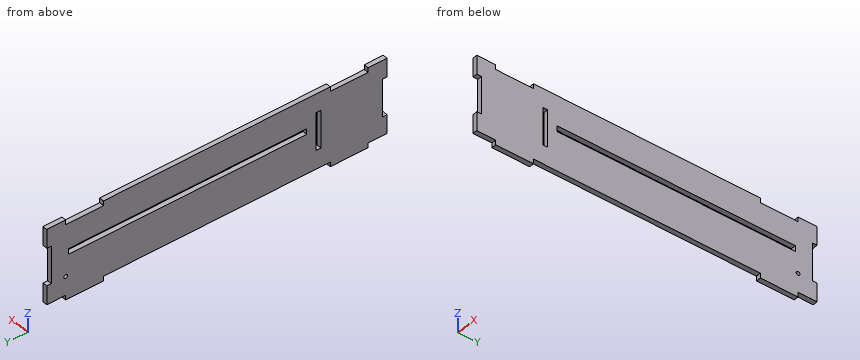
from build123d import *

# Parameters (mm, degrees)
F0_W      = 457.2
F0_H      = 101.6
F1_DEPTH  = 6.35
F2_W      = 50.8
F2_H      = 6.35
F3_DEPTH  = 6.35
F4_R      = 2.54
F5_DEPTH  = 6.351
F6_W      = 6.35
F6_H      = 50.8
F7_DEPTH  = 25.4
F9_W      = 6.35
F9_H      = 50.8
F10_DEPTH = 25.4
F11_W     = 50.8
F11_H     = 6.35
F12_DEPTH = 25.4
F13_W     = 320.04
F13_H     = 7.62
F14_DEPTH = 25.4


with BuildPart() as f1:
    # F0 (on Right) → F1 (new body)
    with BuildSketch(Plane.YZ):
        with Locations((0, 50.8)):
            Rectangle(F0_W, F0_H)
    extrude(amount=F1_DEPTH)

    # F4 (on face) → F5 (cut, through all)
    with BuildSketch(Plane.YZ.offset(6.35)):
        with Locations((203.2, 25.4)):
            Circle(F4_R)
    extrude(amount=-F5_DEPTH, mode=Mode.SUBTRACT)

    # F6 (on face) → F7 (cut)
    with BuildSketch(Plane.YZ.offset(6.35)):
        with Locations((225.425, 50.8)):
            Rectangle(F6_W, F6_H)
        with Locations((-225.425, 50.8)):
            Rectangle(F6_W, F6_H)
    extrude(amount=-F7_DEPTH, mode=Mode.SUBTRACT)


with BuildPart() as f3:
    # F2 (on face) → F3 (new body)
    with BuildSketch(Plane.YZ.offset(6.35)):
        with Locations((177.8, -3.175)):
            Rectangle(F2_W, F2_H)
        with Locations((-177.8, -3.175)):
            Rectangle(F2_W, F2_H)
    extrude(amount=-F3_DEPTH)

    # F8: union F1
    add(f1.part)

    # F9 (on face) → F10 (cut)
    with BuildSketch(Plane.YZ.offset(6.35)):
        with Locations((-136.525, 50.8)):
            Rectangle(F9_W, F9_H)
    extrude(amount=-F10_DEPTH, mode=Mode.SUBTRACT)

    # F11 (on face) → F12 (cut)
    with BuildSketch(Plane.YZ.offset(6.35)):
        with Locations((-177.8, 98.425)):
            Rectangle(F11_W, F11_H)
        with Locations((177.8, 98.425)):
            Rectangle(F11_W, F11_H)
    extrude(amount=-F12_DEPTH, mode=Mode.SUBTRACT)

    # F13 (on face) → F14 (cut)
    with BuildSketch(Plane.YZ.offset(6.35)):
        with Locations((39.37, 57.15)):
            Rectangle(F13_W, F13_H)
    extrude(amount=-F14_DEPTH, mode=Mode.SUBTRACT)


solid = f3.part
The model under review builds one solid part; all positions refer to its coordinate system, in mm. Round coordinates to 2 decimals unless told otherwise and drop trailing zeros. Write each loop counter-clockwise with the first axis right and the second up, starting at its lowest first coordinate (ties: lowest second). Pieces come first, ordered by that corner, then holes. Notation, with made-up numbers: M -34,67 L 25,67 A29 ccw 25,87 Z; hole C 2.5,-24 d2. An arc over 180 degrees is marked long. Use a Markdown table: item, result. Add a question column.
Q1. We need section B-B, the plane z = 67. State the section outline as (x, y) points.
Q2. We need section C-C, the plane x = 1. Count the separate pieces of the cut face and the enclosed holes in it, plus the area to 3 significant figures.
Q3. Insertion check: pin 1 (1.9 mm diameter, centred on x = 4, z = -4, fed in from +Y); pin 2 (3 mm diameter, centred on x = 2, y = -219, fed in from -Z); pin 3 (1 mm diameter, centred on x = 1, z = 57.5, fed in from -Y). Each pin has a flat end and moves straight along its axis. Give the tip position at first contact, or say it passes through.
Q4. We need section A-A, the plane y = -96. State the section outline as (x, z) points.
Q5. To check wall thickness, follow line 1 (Y direction, x = 1, z = 48.5); line 2 (Z direction, x = 2.25, y = 90); line 3 (Y direction, x = 1.25, z = -0.5). State the ranges of each line that lie inside material, in increasing order.
Findings below:
| question | item | result |
|---|---|---|
| 1 | outline | M 0,-222.25 L 6.35,-222.25 L 6.35,-139.7 L 0,-139.7 Z; M 0,-133.35 L 6.35,-133.35 L 6.35,222.25 L 0,222.25 Z |
| 2 | separate pieces | 1 |
| 2 | enclosed holes | 3 |
| 2 | area | 43,000 mm² |
| 3 | pin 1 | stops at y = 203.2 |
| 3 | pin 2 | stops at z = 0 |
| 3 | pin 3 | stops at y = -222.25 |
| 4 | outline | M 0,0 L 6.35,0 L 6.35,53.34 L 0,53.34 Z; M 0,60.96 L 6.35,60.96 L 6.35,101.6 L 0,101.6 Z |
| 5 | line 1 | y = -222.25 to -139.7, -133.35 to 222.25 |
| 5 | line 2 | z = 0 to 53.34, 60.96 to 101.6 |
| 5 | line 3 | y = -203.2 to -152.4, 152.4 to 203.2 |
